CAD build for the part. Positions are in the model's coordinates, mm. A direction names the side the tool comes from. Round coordinates to 2 decimals unless told otherwise and drop trailing zeros. Order: outer loops, then holes, each group sorted by start corner. A loop starts at its lowest first (then second) coordinate and runs counter-clockwise, first axis right, second up.
```python
from build123d import *

# Parameters (mm, degrees)
SKETCH1_W           = 40
SKETCH1_H           = 250
BOSS_EXTRUDE1_DEPTH = 20
SKETCH2_W           = 40
SKETCH2_H           = 75
CUT_EXTRUDE1_DEPTH  = 10
FILLET1_R           = 10
SKETCH3_R           = 10
CUT_EXTRUDE2_DEPTH  = 10
SKETCH5_W           = 20
SKETCH5_H           = 40
BOSS_EXTRUDE2_DEPTH = 150
FILLET2_R           = 10
FILLET3_R           = 10


with BuildPart() as part:
    # Sketch1 → Boss-Extrude1 (new body)
    with BuildSketch(Plane(origin=(0, 0, 0), x_dir=(0, 0, -1), z_dir=(1, 0, 0))):
        Rectangle(SKETCH1_W, SKETCH1_H)
    extrude(amount=BOSS_EXTRUDE1_DEPTH)

    # Sketch2 → Cut-Extrude1 (cut)
    with BuildSketch(Plane.ZY):
        with Locations((0, 87.5)):
            Rectangle(SKETCH2_W, SKETCH2_H)
    extrude(amount=-CUT_EXTRUDE1_DEPTH, mode=Mode.SUBTRACT)

    # Fillet1
    fillet1_edges = [part.edges().sort_by_distance(p)[0] for p in [
        (15, 125, 20),
        (15, 125, -20),
    ]]
    fillet(fillet1_edges, radius=FILLET1_R)

    # Sketch3 → Cut-Extrude2 (cut)
    with BuildSketch(Plane(origin=(20, 0, 0), x_dir=(0, 0, -1), z_dir=(1, 0, 0))):
        with Locations((0, 105)):
            Circle(SKETCH3_R)
    extrude(amount=-CUT_EXTRUDE2_DEPTH, mode=Mode.SUBTRACT)

    # Sketch5 → Boss-Extrude2 (add)
    with BuildSketch(Plane(origin=(0, 0, -20), x_dir=(-1, 0, 0), z_dir=(0, 0, -1))):
        with Locations((-10, -145)):
            Rectangle(SKETCH5_W, SKETCH5_H)
    extrude(amount=-BOSS_EXTRUDE2_DEPTH)

    # Fillet2
    fillet2_edges = [part.edges().sort_by_distance(p)[0] for p in [
        (10, -165, -20),
    ]]
    fillet(fillet2_edges, radius=FILLET2_R)

    # Fillet3
    fillet3_edges = [part.edges().sort_by_distance(p)[0] for p in [
        (10, -125, 20),
    ]]
    fillet(fillet3_edges, radius=FILLET3_R)


solid = part.part
```
1. Cut at B-B, the plane y = 105. Write the cut outline in (x, z).
2. Mould opens along Z. For faces 1 (the face through (10, -18, -20)), 2 (the face through (15.07, 114.915, 1.302)), 3 (the face through (20, -53, 16)) say: released by +Z, released by -Z, zero draft, split by the parting line, or undercut.
3. Cut at D-D, the plane y = -28. Write the cut outline in (x, z), and give its area (3 significant figures).
4. Cut at C-C, the plane z = 59.5. Write the cut outline in (x, y).
5. Cut at A-A, the plane z = 0. Write the cut outline in (x, y), and give its area (3 significant figures).
6. Drill centre lines: line 1 (Y direction, x = 12, z = 0); line 2 (Z direction, x = 6.25, y = 7); line 3 (Y direction, x = 16.25, z = 108). Where is each one in solid material? Low to high.
7. Pin check, flat tips, straight feed: P1, Ø1.5, axis at x = 5, y = -118.5, coming from the +Z side; P2, Ø10, axis at x = 12, z = 86.5, coming from the +Y side; P3, Ø8, axis at x = 5.5, z = 10, coming from the +Y side. Stop position of each tip, or through.
8. Tool access for faces 4 (the face through (10, 88, 0)), 5 (the face through (10, -165, 59)), 6 (the face through (10, -125, 79)): list every direction of +Z, -Z, +X, -X, +Y, -Y with a clear straight run to the whole face (end or side of a thin tool).
Outcome:
1. outline: (10, -20) - (20, -20) - (20, -10) - (10, -10) - close; (10, 10) - (20, 10) - (20, 20) - (10, 20) - close
2. face 1: released by -Z
2. face 2: undercut
2. face 3: zero draft
3. outline: (0, -20) - (20, -20) - (20, 20) - (0, 20) - close
3. area: 800 mm2
4. outline: (0, -165) - (20, -165) - (20, -125) - (0, -125) - close
5. outline: (0, -165) - (20, -165) - (20, 95) - (10, 95) - (10, 50) - (0, 50) - close; (10, 115) - (20, 115) - (20, 125) - (10, 125) - close
5. area: 4,850 mm2
6. line 1: y = -165 to 95, 115 to 125
6. line 2: z = -20 to 20
6. line 3: y = -165 to -125
7. P1: stops at z = 20.95
7. P2: stops at y = -125
7. P3: stops at y = 50
8. face 4: +Z, -Z, -X, +Y
8. face 5: +Z, -Z, +X, -X, -Y
8. face 6: +Z, +X, -X, +Y
